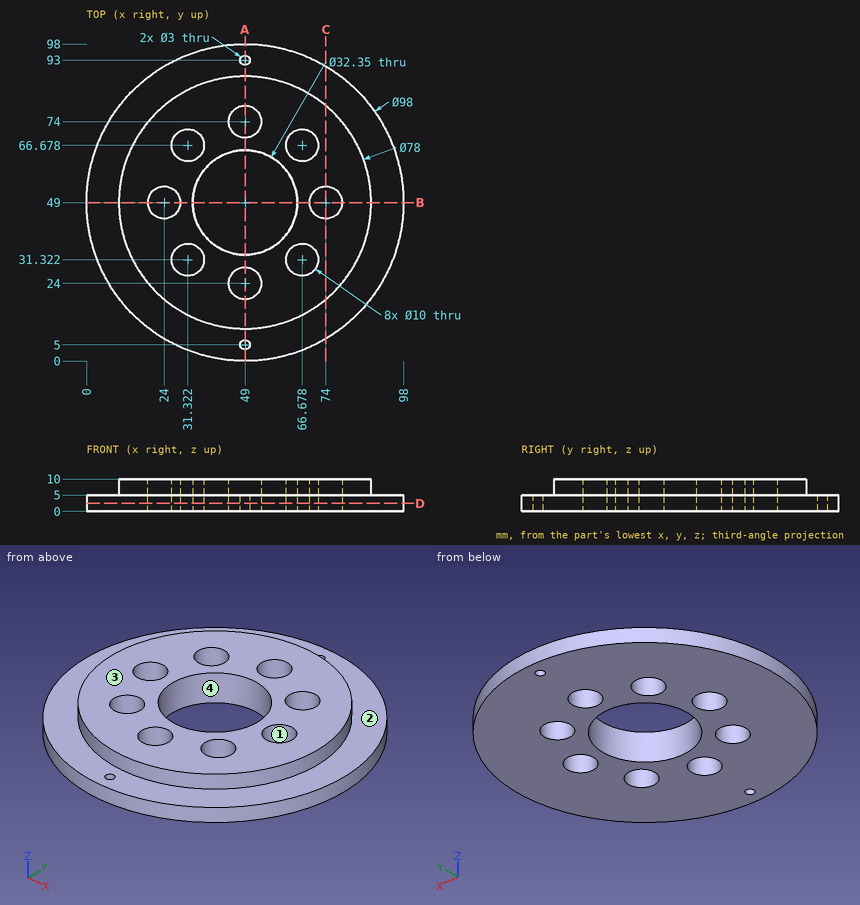
For this review, use the dimensioned drawing (mm, ordinates from the lowest corner) and the shaded views. A direction names the side the tool comes from. Give positions to 0.01 mm unless a question says otherwise; leave off trailing zeros. Order: outer loops, then holes, each group sorted by start corner. A loop starts at its lowest first (then second) coordinate and runs counter-clockwise, first axis right, second up. Notation, with made-up numbers: (56, 84.5) - (82, 84.5) arc R19 cw to (82, 94.5) - close; hole circle Ø5 at (-24.5, 38.25). An arc over 180 degrees is marked (long way). Use CSV: the item, a comma, the result in double quotes. Start each with the question number.
Q1. For line 1 (X direction, y = 51, z = 6.5); line 2 (Y direction, x = 75, z = 6.25); line 3 (X direction, y = 59.5, z = 4.75) (1 decimal), list the stretches that pass through material, from the lowest coordinate up.
Q2. Machinability: for the marked faces 1 and 2, which of the approach directions +Z, -Z, +X, -X, +Y, -Y give a long, thin tool a straight path to every point of the face, cutting with its end or side? Answer none if there is none.
Q3. Take a section at B-B (y = 49). State the section outline as (x, z) points (1 decimal).
Q4. For P1, Ø3, axis at x = 73, y = 47.5, coming from the -Z side; P2, Ø5, axis at x = 74, z = 1.5, coming from the +Y side; P3, Ø2, axis at x = 28.5, z = 4, coming from the -Y side; P4, Ø2, axis at y = 45.5, z = 3, coming from the -X side, all flat-tipped, find the tip position at first contact; note any pin that passes through.
Q5. Take a section at C-C (x = 74). State the section outline as (y, z) points.
Q6. Take a section at D-D (z = 2.5). Count the separate pieces of the cut face and the enclosed holes in it, and give its area (3 significant figures).
Q7. Take a section at A-A (x = 49). State the section outline as (y, z) points (1 decimal).
Q8. Draft analysis for pull direction Y (two halves, no side actions). For the marked faces 3 and 4, state which applies: pulls with the +Y half, pulls with the -Y half, needs draft (parallel to the pull), parting line crosses it, or undercut.
Calculated:
1,line 1,"x = 10.05 to 19.42, 28.58 to 32.95, 65.05 to 69.42, 78.58 to 87.95"
1,line 2,"y = 19.93 to 44.1, 53.9 to 78.07"
1,line 3,"x = 1.1 to 36.7, 61.3 to 96.9"
2,face 1,"+Z, -Z"
2,face 2,"+Z"
3,outline,"(0, 0) - (19, 0) - (19, 10) - (10, 10) - (10, 5) - (0, 5) - close; (29, 0) - (32.8, 0) - (32.8, 10) - (29, 10) - close; (65.2, 0) - (69, 0) - (69, 10) - (65.2, 10) - close; (79, 0) - (98, 0) - (98, 5) - (88, 5) - (88, 10) - (79, 10) - close"
4,P1,"passes through"
4,P2,"stops at y = 92.53"
4,P3,"stops at y = 4.05"
4,P4,"stops at x = 0.06"
5,outline,"(6.86, 0) - (44, 0) - (44, 10) - (19.07, 10) - (19.07, 5) - (6.86, 5) - close; (54, 0) - (91.14, 0) - (91.14, 5) - (78.93, 5) - (78.93, 10) - (54, 10) - close"
6,separate pieces,"1"
6,enclosed holes,"11"
6,area,"6,080 mm²"
7,outline,"(0, 0) - (3.5, 0) - (3.5, 5) - (0, 5) - close; (6.5, 0) - (19, 0) - (19, 10) - (10, 10) - (10, 5) - (6.5, 5) - close; (29, 0) - (32.8, 0) - (32.8, 10) - (29, 10) - close; (65.2, 0) - (69, 0) - (69, 10) - (65.2, 10) - close; (79, 0) - (91.5, 0) - (91.5, 5) - (88, 5) - (88, 10) - (79, 10) - close; (94.5, 0) - (98, 0) - (98, 5) - (94.5, 5) - close"
8,face 3,"needs draft"
8,face 4,"undercut"
